from build123d import *

# Parameters (mm, degrees)
F1_DEPTH = 6.985
F2_R     = 1.27
F3_R     = 1.27


with BuildPart() as f1:
    # F0 (on Top) → F1 (new body)
    with BuildSketch(Plane.XY):
        with BuildLine():
            Line((15.71625, 9.0737811682), (13.7528333371, 7.9402020293))
            ThreePointArc((13.7528333371, 7.9402020293), (15.3392924121, 4.1101510143), (15.8804040586, 0))
            ThreePointArc((15.8804040586, 0), (15.3392924121, -4.1101510143), (13.7528333371, -7.9402020293))
            Line((13.7528333371, -7.9402020293), (15.71625, -9.0737811682))
            Line((15.71625, -9.0737811682), (20.955, 0))
            Line((20.955, 0), (15.71625, 9.0737811682))
        make_face()
        with BuildLine():
            ThreePointArc((0, 15.8804040586), (7.9402020293, 13.7528333371), (13.7528333371, 7.9402020293))
            Line((13.7528333371, 7.9402020293), (15.71625, 9.0737811682))
            Line((15.71625, 9.0737811682), (10.4775, 18.1475623363))
            Line((10.4775, 18.1475623363), (0, 18.1475623363))
            Line((0, 18.1475623363), (0, 15.8804040586))
        make_face()
        with BuildLine():
            Line((15.71625, -9.0737811682), (13.7528333371, -7.9402020293))
            ThreePointArc((13.7528333371, -7.9402020293), (7.9402020293, -13.7528333371), (0, -15.8804040586))
            Line((0, -15.8804040586), (0, -18.1475623363))
            Line((0, -18.1475623363), (10.4775, -18.1475623363))
            Line((10.4775, -18.1475623363), (15.71625, -9.0737811682))
        make_face()
        with BuildLine():
            ThreePointArc((-13.7528333371, 7.9402020293), (-7.9402020293, 13.7528333371), (0, 15.8804040586))
            Line((0, 15.8804040586), (0, 18.1475623363))
            Line((0, 18.1475623363), (-10.4775, 18.1475623363))
            Line((-10.4775, 18.1475623363), (-15.71625, 9.0737811682))
            Line((-15.71625, 9.0737811682), (-13.7528333371, 7.9402020293))
        make_face()
        Polygon((10.4775, 18.1475623363), (15.71625, 9.0737811682), (43.9940905122, 25.4), align=None)
        Polygon((43.9940905122, 25.4), (15.71625, 9.0737811682), (20.955, 0), align=None)
        with BuildLine():
            Line((0, -18.1475623363), (0, -15.8804040586))
            ThreePointArc((0, -15.8804040586), (-7.9402020293, -13.7528333371), (-13.7528333371, -7.9402020293))
            Line((-13.7528333371, -7.9402020293), (-15.71625, -9.0737811682))
            Line((-15.71625, -9.0737811682), (-10.4775, -18.1475623363))
            Line((-10.4775, -18.1475623363), (0, -18.1475623363))
        make_face()
        Polygon((20.955, 0), (15.71625, -9.0737811682), (43.9940905122, -25.4), align=None)
        Polygon((43.9940905122, -25.4), (15.71625, -9.0737811682), (10.4775, -18.1475623363), align=None)
        with BuildLine():
            ThreePointArc((-13.7528333371, -7.9402020293), (-15.8804040586, 0), (-13.7528333371, 7.9402020293))
            Line((-13.7528333371, 7.9402020293), (-15.71625, 9.0737811682))
            Line((-15.71625, 9.0737811682), (-20.955, 0))
            Line((-20.955, 0), (-15.71625, -9.0737811682))
            Line((-15.71625, -9.0737811682), (-13.7528333371, -7.9402020293))
        make_face()
        Polygon((-10.4775, 18.1475623363), (0, 18.1475623363), (0, 50.8), align=None)
        Polygon((0, 50.8), (0, 18.1475623363), (10.4775, 18.1475623363), align=None)
        Polygon((10.4775, -18.1475623363), (0, -18.1475623363), (0, -50.8), align=None)
        Polygon((0, -50.8), (0, -18.1475623363), (-10.4775, -18.1475623363), align=None)
        Polygon((-20.955, 0), (-15.71625, 9.0737811682), (-43.9940905122, 25.4), align=None)
        Polygon((-43.9940905122, 25.4), (-15.71625, 9.0737811682), (-10.4775, 18.1475623363), align=None)
        Polygon((-10.4775, -18.1475623363), (-15.71625, -9.0737811682), (-43.9940905122, -25.4), align=None)
        Polygon((-43.9940905122, -25.4), (-15.71625, -9.0737811682), (-20.955, 0), align=None)
        with BuildLine():
            ThreePointArc((-9.5357191185, 5.50545), (-5.50545, 9.5357191185), (0, 11.0109))
            Line((0, 11.0109), (0, 15.8804040586))
            ThreePointArc((0, 15.8804040586), (-7.9402020293, 13.7528333371), (-13.7528333371, 7.9402020293))
            Line((-13.7528333371, 7.9402020293), (-9.5357191185, 5.50545))
        make_face()
        with BuildLine():
            ThreePointArc((0, 11.0109), (5.50545, 9.5357191185), (9.5357191185, 5.50545))
            Line((9.5357191185, 5.50545), (13.7528333371, 7.9402020293))
            ThreePointArc((13.7528333371, 7.9402020293), (7.9402020293, 13.7528333371), (0, 15.8804040586))
            Line((0, 15.8804040586), (0, 11.0109))
        make_face()
        with BuildLine():
            ThreePointArc((9.5357191185, 5.50545), (10.6357126807, 2.8498306237), (11.0109, 0))
            ThreePointArc((11.0109, 0), (10.6357126807, -2.8498306237), (9.5357191185, -5.50545))
            Line((9.5357191185, -5.50545), (13.7528333371, -7.9402020293))
            ThreePointArc((13.7528333371, -7.9402020293), (15.3392924121, -4.1101510143), (15.8804040586, 0))
            ThreePointArc((15.8804040586, 0), (15.3392924121, 4.1101510143), (13.7528333371, 7.9402020293))
            Line((13.7528333371, 7.9402020293), (9.5357191185, 5.50545))
        make_face()
        with BuildLine():
            Line((13.7528333371, -7.9402020293), (9.5357191185, -5.50545))
            ThreePointArc((9.5357191185, -5.50545), (5.50545, -9.5357191185), (0, -11.0109))
            Line((0, -11.0109), (0, -15.8804040586))
            ThreePointArc((0, -15.8804040586), (7.9402020293, -13.7528333371), (13.7528333371, -7.9402020293))
        make_face()
        with BuildLine():
            Line((0, -15.8804040586), (0, -11.0109))
            ThreePointArc((0, -11.0109), (-5.50545, -9.5357191185), (-9.5357191185, -5.50545))
            Line((-9.5357191185, -5.50545), (-13.7528333371, -7.9402020293))
            ThreePointArc((-13.7528333371, -7.9402020293), (-7.9402020293, -13.7528333371), (0, -15.8804040586))
        make_face()
        with BuildLine():
            ThreePointArc((-9.5357191185, -5.50545), (-11.0109, 0), (-9.5357191185, 5.50545))
            Line((-9.5357191185, 5.50545), (-13.7528333371, 7.9402020293))
            ThreePointArc((-13.7528333371, 7.9402020293), (-15.8804040586, 0), (-13.7528333371, -7.9402020293))
            Line((-13.7528333371, -7.9402020293), (-9.5357191185, -5.50545))
        make_face()
    extrude(amount=F1_DEPTH)

    # F2
    f2_edges = [f1.edges().sort_by_distance(p)[0] for p in [
        (0, 50.8, 3.4925),
        (-43.994091, -25.4, 3.4925),
        (-43.994091, 25.4, 3.4925),
        (0, -50.8, 3.4925),
        (43.994091, -25.4, 3.4925),
        (43.994091, 25.4, 3.4925),
    ]]
    fillet(f2_edges, radius=F2_R)

    # F3
    f3_edges = [f1.edges().sort_by_distance(p)[0] for p in [
        (31.145007, -11.234219, 6.985),
        (5.843385, -32.589477, 6.985),
        (-25.301622, -21.355258, 6.985),
        (-31.145007, 11.234219, 6.985),
        (25.301622, 21.355258, 6.985),
        (-5.843385, 32.589477, 6.985),
        (25.301622, 21.355258, 0),
        (25.301622, -21.355258, 0),
        (5.843385, -32.589477, 0),
        (-25.301622, -21.355258, 0),
        (-31.145007, 11.234219, 0),
        (5.843385, 32.589477, 0),
    ]]
    fillet(f3_edges, radius=F3_R)


solid = f1.part
For this review, take the finished solid that the model builds, in its own axes (mm). A direction names the side the tool comes from. Give positions to 0.01 mm unless a question says otherwise; leave off trailing zeros. Loops run counter-clockwise (first coordinate to the right, second up) from the corner with the lowest first, then second, coordinate; pieces in that order, holes last. Notation, with made-up numbers: M 89.5,3 L 106.5,3 A21 cw 106.5,24 Z; hole C -1.75,52 d10. An arc over 180 degrees is marked long. Answer as a JSON object with one key per item and string values. Group by question number.
Q1. Mouldability with a two-part tool opening along Y and no side actions: class faces 6 (the flat face through (-5.908, -32.387, 3.461)), 7 (the flat face through (-31.002, -11.077, 3.461)), 8 (the cylindrical face through (-5.72, 31.71, 0.36)) as +Y half, -Y half, draft (parallel to the pull), parting line (faces both ways), or undercut.
Q2. Add section A-A on z = 3.25. Give the boundary of the cut face in (x, y) (1 decimal).
Q3. Tool access review of faces 1 (the cylindrical face through (5.72, -31.71, 0.36)), 2 (the flat face through (25.09, -21.31, 3.46)), 3 (the cylindrical face through (24.6, 20.81, 0.36)), 4 (the cylindrical face through (-30.64, -11.21, 6.6)), 5 (the cylindrical face through (-5.59, -32.13, 6.62)): name each direction out of +Z, -Z, +X, -X, +Y, -Y from which nothing blocks a thin tool from reaching the whole face with its end or side.
Q4. Insertion check: P1, Ø1, axis at y = 34.5, z = 4, coming from the +X side; P2, Ø3, axis at y = -35, z = 4, coming from the -X side. Each pin has a flat end and moves straight along its axis. Give the tip position at first contact, or say it passes through.
Q5. For probe 1 along Y at (x, z) = (37.5, 3.75); probe 2 along X at (y, z) = (33.5, 1); probe 3 along X at (y, z) = (7, 5.5), list the stretches that pass through material, from the lowest coordinate up. Write a range as [from, to].
Checked values:
{
 "1": {"face 6": "-Y half", "face 7": "undercut", "face 8": "+Y half"},
 "2": {"outline": "M -41.3,-22.5 A1.3 ccw -40.1,-24.6 L -10.5,-18.1 L -1.2,-47 A1.3 ccw 1.2,-47 L 10.5,-18.1 L 40.1,-24.6 A1.3 ccw 41.3,-22.5 L 21,0 L 41.3,22.5 A1.3 ccw 40.1,24.6 L 10.5,18.1 L 1.2,47 A1.3 ccw -1.2,47 L -10.5,18.1 L -40.1,24.6 A1.3 ccw -41.3,22.5 L -21,0 Z; hole C 0,0 d22"},
 "3": {"face 1": "-Z, -Y", "face 2": "+Z, -Z, -Y", "face 3": "-Z, +Y", "face 4": "+Z, -X", "face 5": "+Z, -Y"},
 "4": {"P1": "x = 5.39", "P2": "x = -5.55"},
 "5": {"probe 1": "[-23.99, -18.24], [18.24, 23.99]", "probe 2": "[-5.52, 5.52]", "probe 3": "[-27.3, -8.5], [8.5, 27.3]"}
}
